Geometry: final body of the model. Coordinates: model frame, mm. A direction names the side the tool comes from. Round coordinates to 2 decimals unless told otherwise and drop trailing zeros. Loops run counter-clockwise (first coordinate to the right, second up) from the corner with the lowest first, then second, coordinate; pieces in that order, holes last. Notation, with made-up numbers: M 56,30 L 93,30 A21 ccw 93,39 Z; hole C 52.5,45 d1. An arc over 180 degrees is marked long. Return JSON: item names as keys, results as strings.
from build123d import *

# Parameters (mm, degrees)
ESBO_O1_R                = 21
ESBO_O1_R_2              = 3.1
RESSALTO_EXTRUS_O1_DEPTH = 5
ESBO_O3_R                = 7.5
CORTE_EXTRUS_O1_DEPTH    = 19


with BuildPart() as part:
    # Esboço1 → Ressalto-extrusão1 (new body)
    with BuildSketch(Plane.XY):
        with BuildLine():
            ThreePointArc((26.22105388, -15.579035061), (0, 30.5), (-26.22105388, -15.579035061))
            ThreePointArc((-26.22105388, -15.579035061), (-26.087819075, -16.82024855), (-26.940019837, -17.73245264))
            ThreePointArc((-26.940019837, -17.73245264), (-28.794642857, -25.856499042), (-20.518582449, -24.883575301))
            ThreePointArc((-20.518582449, -24.883575301), (-19.520268693, -24.134087419), (-18.30049416, -24.399629372))
            ThreePointArc((-18.30049416, -24.399629372), (0, -30.5), (18.30049416, -24.399629372))
            ThreePointArc((18.30049416, -24.399629372), (19.520268693, -24.134087419), (20.518582449, -24.883575301))
            ThreePointArc((20.518582449, -24.883575301), (28.794642857, -25.856499042), (26.940019837, -17.73245264))
            ThreePointArc((26.940019837, -17.73245264), (26.087819075, -16.82024855), (26.22105388, -15.579035061))
        make_face()
        Circle(ESBO_O1_R, mode=Mode.SUBTRACT)
        with Locations((25, -22.449053432)):
            Circle(ESBO_O1_R_2, mode=Mode.SUBTRACT)
        with Locations((-25, -22.449053432)):
            Circle(ESBO_O1_R_2, mode=Mode.SUBTRACT)
    extrude(amount=RESSALTO_EXTRUS_O1_DEPTH)

    # Esboço2 → Revolução1 (revolve)
    with BuildSketch(Plane(origin=(0, 0, 0), x_dir=(1, 0, 0), z_dir=(0, 1, 0))):
        Polygon((30.5, 0), (3.175, 19.133170982), (3.175, 39.133170982), (1.675, 39.133170982), (1.675, 13.531510676), (21, 0), align=None)
    revolve(axis=Axis((0, 0, 0), (0, 0, -1)))

    # Esboço3 → Corte-extrusão1 (cut)
    with BuildSketch(Plane(origin=(0, 0, 0), x_dir=(-1, 0, 0), z_dir=(0, 0, -1))):
        with Locations((-25, -22.449053432)):
            Circle(ESBO_O3_R)
        with Locations((25, -22.449053432)):
            Circle(ESBO_O3_R)
    extrude(amount=CORTE_EXTRUS_O1_DEPTH, mode=Mode.SUBTRACT)


solid = part.part
Q1. Section query A-A (x = 0). Output: boundary loops of the cut face in (y, z) (3 decimals), plus the area to 3 significant figures.
Determined:
{"outline": "M -30.5,0 L -3.175,-19.133 L -3.175,-39.133 L -1.675,-39.133 L -1.675,-13.532 L -21,0 L -21,5 L -30.5,5 Z; M 1.675,-39.133 L 3.175,-39.133 L 3.175,-19.133 L 30.5,0 L 30.5,5 L 21,5 L 21,0 L 1.675,-13.532 Z", "area": "474 mm^2"}
Q2. Pull-direction query (Y, two-part tool) for faces 1 (the cylindrical face through (28.7, -25.96, 2.46)), 2 (the flat face through (-7, -20, 5)), 3 (the cylindrical face through (19.5, -24.13, 2.46)); classes: pulls with the +Y half, pulls with the -Y half, needs draft (parallel to the pull), parting line crosses it, or undercut.
Determined:
{"face 1": "undercut", "face 2": "needs draft", "face 3": "pulls with the -Y half"}
Q3. Reachability of faces 4 (the cylindrical face through (-0.69, 3.1, -29.27)), 5 (the cylindrical face through (20.03, 6.31, 2.46)), 6 (the cylindrical face through (-25.672, -25.475, 2.465)) from +Z, -Z, +X, -X, +Y, -Y: full face, straight path, thin tool, end or side. Return the list, or none.
Determined:
{"face 4": "-Z", "face 5": "+Z", "face 6": "+Z, -Z"}
Q4. Pin query (flat end, axial travel): pin 1 (2 mm diameter, centred on y = 7.5, z = -13.5, fed in from +X); pin 2 (1.5 mm diameter, centred on x = 14, z = -3, fed in from -Y); pin 3 (10 mm diameter, centred on x = 21, y = -24.5, fed in from -Z). Return the tip coordinate at first contact, or that it passes through.
Determined:
{"pin 1": "stops at x = 10.32", "pin 2": "stops at y = -23.5", "pin 3": "stops at z = -2.26"}
Q5. Material intervals for L1, parallel to Y at x = 0, z = -22.5 (3 decimals); L2, parallel to X at y = -26.5, z = 1, sorted ascending.
Determined:
{"L1": "y = -3.175 to -1.675, 1.675 to 3.175", "L2": "x = -28.1 to -21.9, -15.1 to 15.1, 21.9 to 28.1"}
Q6. Section query C-C (z = -32.5). Output: boundary loops of the cut face in (x, y) (3 decimals), plus the area to 3 significant figures.
Determined:
{"outline": "C 0,0 d6.35; hole C 0,0 d3.35", "area": "22.9 mm^2"}
Q7. Section query D-D (z = -8). Output: boundary loops of the cut face in (x, y).
Determined:
{"outline": "C 0,0 d38.15; hole C 0,0 d19.15"}
